Input: part model. Units: mm. Frame: model coordinates. Face numbers are marked on the shaded views. Coordinates: 2 decimals unless noted, no trailing zeros. Order: outer loops, then holes, each group sorted by start corner. A loop starts at its lowest first (then second) coordinate and runs counter-clockwise, first axis right, second up. Notation, with made-up numbers: (-3, 79) - (18, 79) arc R15 cw to (18, 87) - close; hole circle Ø11 at (-30, 44). An arc over 180 degrees is marked (long way). One line per question, with ' | ' between items.
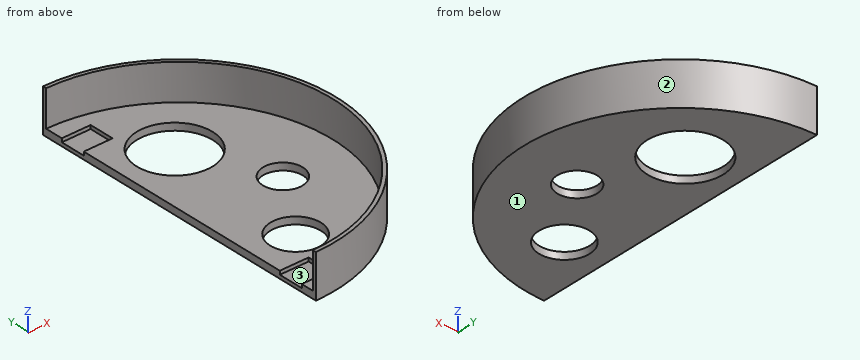
from build123d import *

# Parameters (mm, degrees)
F1_DEPTH = 12
F2_R     = 42.5
F3_DEPTH = 10
F4_R     = 10.5
F4_R_2   = 5.5
F4_R_3   = 7
F5_DEPTH = 2.001
F6_W     = 7
F6_H     = 1
F7_DEPTH = 8


with BuildPart() as f1:
    # F0 (on Top) → F1 (new body)
    with BuildSketch(Plane.XY):
        with BuildLine():
            Line((0, 43.5), (0, -43.5))
            ThreePointArc((0, -43.5), (43.5, 0), (0, 43.5))
        make_face()
    extrude(amount=F1_DEPTH)

    # F2 (on face) → F3 (cut)
    with BuildSketch(Plane.XY.offset(12)):
        Circle(F2_R)
    extrude(amount=-F3_DEPTH, mode=Mode.SUBTRACT)

    # F4 (on face) → F5 (cut, through all)
    with BuildSketch(Plane.XY.offset(2)):
        with Locations((-15, 18.734994)):
            Circle(F4_R)
        with Locations((-25, -4.265006)):
            Circle(F4_R_2)
        with Locations((-12, -23.265006)):
            Circle(F4_R_3)
        with Locations((15, 18.734994)):
            Circle(F4_R)
        with Locations((25, -4.265006)):
            Circle(F4_R_2)
        with Locations((12, -23.265006)):
            Circle(F4_R_3)
    extrude(amount=-F5_DEPTH, mode=Mode.SUBTRACT)

    # F6 (on face) → F7 (cut)
    with BuildSketch(Plane(origin=(0, 0, 0), x_dir=(0, -1, 0), z_dir=(-1, 0, 0))):
        with Locations((-34, 1.5)):
            Rectangle(F6_W, F6_H)
        with Locations((35.5, 1.5)):
            Rectangle(F6_W, F6_H)
    extrude(amount=-F7_DEPTH, mode=Mode.SUBTRACT)


solid = f1.part
Item 1: Ray query, line 1 (Y direction, x = 12, z = 1.4) (3 decimals); line 2 (Z direction, x = 16, y = -38.5); line 3 (Y direction, x = 19, z = 5.5). Return the intervals inside material, ascending.
Data:
line 1: -41.812 to -30.265, -16.265 to 8.673, 28.797 to 41.812 | line 2: 0 to 2 | line 3: -39.13 to -38.02, 38.02 to 39.13
Item 2: Section A-A on x = 12. Return the cut outline in (y, z) (3 decimals), and give its area (3 significant figures).
Data:
outline: (-41.812, 0) - (-30.265, 0) - (-30.265, 2) - (-40.771, 2) - (-40.771, 12) - (-41.812, 12) - close; (-16.265, 0) - (8.673, 0) - (8.673, 2) - (-16.265, 2) - close; (28.797, 0) - (41.812, 0) - (41.812, 12) - (40.771, 12) - (40.771, 2) - (28.797, 2) - close | area: 120 mm^2
Item 3: Contact query for flat-ended pins moving along their axis: P1, Ø5.5, axis at x = 4, y = 35.5, coming from the +Z side; P2, Ø0.8, axis at x = 5.5, z = 1.5, coming from the +Y side; P3, Ø5.5, axis at x = 3.5, y = -36, coming from the +Z side; P4, Ø9, axis at x = 25, y = -4.27, coming from the +Z side. Output: stop coordinate, or through.
Data:
P1: z = 2 | P2: y = 43.2 | P3: z = 1 | P4: through
Item 4: Draft query along Y for the marked faces 1, 2 and 3. Return one class per face: released by +Y, released by -Y, zero draft, split by the parting line, or undercut.
Data:
face 1: zero draft | face 2: split by the parting line | face 3: undercut
Item 5: Section D-D on y = 17. Return the cut outline in (x, z), and give its area (3 significant figures).
Data:
outline: (0, 0) - (4.64, 0) - (4.64, 2) - (0, 2) - close; (25.36, 0) - (40.04, 0) - (40.04, 12) - (38.95, 12) - (38.95, 2) - (25.36, 2) - close | area: 49.5 mm^2
Item 6: Section C-C on z = 5.75. Return the cut outline in (x, y), and give its area (3 significant figures).
Data:
outline: (0, -43.5) arc R43.5 ccw to (0, 43.5) - (0, 42.5) arc R42.5 cw to (0, -42.5) - close | area: 135 mm^2
Item 7: Section B-B on y = 0. Return the cut outline in (x, z).
Data:
outline: (0, 0) - (21.53, 0) - (21.53, 2) - (0, 2) - close; (28.47, 0) - (43.5, 0) - (43.5, 12) - (42.5, 12) - (42.5, 2) - (28.47, 2) - close
